Solid Edge part; units mm, degrees
sketch "Sketch1" plane through (0, 0, 0) normal (0, 0, 1) x (1, 0, 0)
  line L0 (23.094, -40) -> (46.188, 0)
  line L1 (46.188, 0) -> (23.094, 40)
  line L2 (23.094, 40) -> (-23.094, 40)
  line L3 (-23.094, 40) -> (-46.188, 0)
  line L4 (-46.188, 0) -> (-23.094, -40)
  line L5 (-23.094, -40) -> (23.094, -40)
  circle A0 centre (0, 0) radius 20
extrude "Protrusion1" add sketch "Sketch1" along normal mid plane 25
sketch "Sketch2" plane through (0, 0, 0) normal (0, -1, 0) x (1, 0, 0)
  line L0 (41.088, 12.5) -> (46.188, 7.4)
  line L1 (46.188, 12.5) -> (46.188, 7.4)
  line L2 (46.188, 12.5) -> (41.088, 12.5)
revolve "RevolvedCutout1" cut sketch "Sketch2" angle 360 about axis through (0, 0, -26.9606) along (0, 0, 1)
Build history of the part. All positions in model axes, mm. Round coordinates to 2 decimals unless told otherwise and drop trailing zeros. Loops run counter-clockwise (first coordinate to the right, second up) from the corner with the lowest first, then second, coordinate; pieces in that order, holes last.
Item 1: Saw through at A-A (x = 0). List the corners of the cut face in (y, z), then the cut area to 3 significant figures.
Item 2: Saw through at C-C (y = -25). List the corners of the cut face in (x, z), then the cut area to 3 significant figures.
Item 3: Pin check, flat tips, straight feed: P1, Ø1.5, axis at y = -26.5, z = -6, coming from the +X side; P2, Ø3, axis at x = 34.5, z = 3, coming from the -Y side; P3, Ø1.5, axis at y = -19, z = 3, coming from the +X side. Stop position of each tip, or through.
Item 4: Two-plate mould, pull along Y, no slides. Class faces 1 (the face through (8.6, 18.3, 12.5)), 2 (the face through (21.42, -36.75, 11.05)), 3 (the face through (-34.48, 20.28, -0.17)), 4 (the face through (-4.336, 19.524, -0.175)): released by +Y, released by -Y, zero draft, split by the parting line, or undercut.
Item 5: Saw through at D-D (x = -33). List the corners of the cut face in (y, z), then the cut area to 3 significant figures.
Item 6: Saw through at B-B (z = 3). List the corners of the cut face in (x, y), then the cut area to 3 significant figures.
Item 7: Drill centre lines: line 1 along X through (y, z) = (-0.5, -5.5); line 2 along Y through (x, z) = (0, -0.25); line 3 along Y through (x, z) = (-7.5, 8.25). Where is each one in solid material? Low to high.
Worked answers:
1. outline: (-40, -12.5) - (-20, -12.5) - (-20, 12.5) - (-40, 12.5) - close; (20, -12.5) - (40, -12.5) - (40, 12.5) - (20, 12.5) - close
1. area: 1,000 mm2
2. outline: (-31.75, -12.5) - (31.75, -12.5) - (31.75, 12.5) - (-31.75, 12.5) - close
2. area: 1,590 mm2
3. P1: stops at x = 31.32
3. P2: stops at y = -22.84
3. P3: stops at x = 35.65
4. face 1: zero draft
4. face 2: released by -Y
4. face 3: released by +Y
4. face 4: undercut
5. outline: (-22.84, -12.5) - (22.84, -12.5) - (22.84, 12.5) - (-22.84, 12.5) - close
5. area: 1,140 mm2
6. outline: (-46.19, 0) - (-23.09, -40) - (23.09, -40) - (46.19, 0) - (23.09, 40) - (-23.09, 40) - close; hole circle Ø40 at (0, 0)
6. area: 4,290 mm2
7. line 1: x = -45.9 to -19.99, 19.99 to 45.9
7. line 2: y = -40 to -20, 20 to 40
7. line 3: y = -40 to -18.54, 18.54 to 40
